Geometry: final body of the model. Coordinates: model frame, mm. A direction names the side the tool comes from. Round coordinates to 2 decimals unless told otherwise and drop trailing zeros. Loops run counter-clockwise (first coordinate to the right, second up) from the corner with the lowest first, then second, coordinate; pieces in that order, holes last. Notation, with made-up numbers: (75.25, 39.5) - (133.25, 39.5) arc R10 ccw to (133.25, 46.5) - close; hole circle Ø5 at (20, -5). An arc over 180 degrees is marked (long way). Return JSON: item names as keys, results as strings. Group by question number.
1. Draft query along X for faces 6 (the face through (20.4, 3.04, 12.43)), 7 (the face through (-6, -9, -17.5)), 8 (the face through (2.1, -14.2, -23.5)). Return one class per face: +X half, -X half, draft (parallel to the pull), parting line (faces both ways), or undercut.
2. Section B-B on z = 26.5. Return loops of the section in (x, y).
3. Material intervals for probe 1 along X at (y, z) = (-14.35, 26.5); probe 2 along X at (y, z) = (0.65, 8); probe 3 along Z at (x, y) = (1, -12), sorted ascending.
4. Section A-A on x = 17.5. Return loops of the section in (y, z).
5. Section C-C on x = 2. Count the separate pieces of the cut face and the enclosed holes in it, and give its area (3 significant figures).
6. First-contact query: pin 1 Ø11.5 at (x, y) = (-21, 15.5) entering from -Z; pin 2 Ø15.5 at (x, z) = (10.5, 2.5) entering from +Y; pin 3 Ø11 at (y, z) = (2.5, -8) entering from -X. Flat tips, straight axial feed; report the tip coordinate or a pass-through.
7. Set-up query: faces 1 (the face through (-6, -6, -20.5)), 2 (the face through (-6, -6, 20.5)), 3 (the face through (-13, 7, 0)), 4 (the face through (-16, -15.25, 26)), 5 (the face through (-31.275, 56.945, 8.709)). Return all of +Z, -Z, +X, -X, +Y, -Y with unobstructed straight access to the full face (end or side cutting, diameter ignored); none if empty.
from build123d import *

# Parameters (mm, degrees)
SKETCH_1_W              = 42
SKETCH_1_H              = 26
SKETCH_1_R              = 1.7
EXTRUDE_1_DEPTH         = 6
SKETCH_15_W             = 6
SKETCH_15_H             = 26
EXTRUDE_4_DEPTH         = 15
EXTRUDE_5_DEPTH         = 26
SKETCH_17_W             = 36
SKETCH_17_H             = 36
SKETCH_17_R             = 1.6
EXTRUDE_6_DEPTH         = 5.638155725
FILLET_3_R              = 2
SKETCH_18_R             = 3
CUT_EXTRUDE_4_DEPTH     = 3
SKETCH_19_R             = 3
CUT_EXTRUDE_5_DEPTH     = 3
FILLET_4_R              = 1
FILLET_6_R              = 5
EXTRUDE_7_DEPTH         = 2
FILLET_7_R              = 5
FILLET_8_R              = 5
SKETCH_21_W             = 30
SKETCH_21_H             = 7.5
EXTRUDE_8_DEPTH         = 6
SKETCH_23_W             = 30
SKETCH_23_H             = 3
EXTRUDE_9_DEPTH         = 17.25
SKETCH_24_W             = 30
SKETCH_24_H             = 4
EXTRUDE_10_DEPTH        = 12
EXTRUDE_11_DEPTH        = 30
FILLET_9_R              = 2
CUT_EXTRUDE_6_DEPTH     = 38
FILLET_11_R             = 2
SKETCH_29_R             = 1.75
CUT_EXTRUDE_7_DEPTH     = 38
SKETCH_30_R             = 3
CUT_EXTRUDE_8_DEPTH     = 2
FILLET_9_OF_MIRROR_2_R  = 2
FILLET_11_OF_MIRROR_2_R = 2
FILLET_14_R             = 2


with BuildPart() as part:
    # 草图1 → 凸台-拉伸1 (new body)
    with BuildSketch(Plane(origin=(0, 0, 0), x_dir=(1, 0, 0), z_dir=(0, 1, 0))):
        Rectangle(SKETCH_1_W, SKETCH_1_H)
        with Locations(Location((17.5, 8, 0), (0, 0, 270))):
            Circle(SKETCH_1_R, mode=Mode.SUBTRACT)
        with Locations(Location((17.5, -8, 0), (0, 0, 90))):
            Circle(SKETCH_1_R, mode=Mode.SUBTRACT)
    extrude(amount=EXTRUDE_1_DEPTH)

    # 草图15 → 凸台-拉伸4 (add)
    with BuildSketch(Plane(origin=(0, 6, 0), x_dir=(1, 0, 0), z_dir=(0, 1, 0))):
        with Locations((-18, 0)):
            Rectangle(SKETCH_15_W, SKETCH_15_H)
    extrude(amount=EXTRUDE_4_DEPTH)

    # 草图16 → 凸台-拉伸5 (add)
    with BuildSketch(Plane.XY.offset(13)):
        Polygon((-15, 21), (-21.858229251, 39.842830003), (-27.15636258, 37.914467174), (-21, 21), align=None)
    extrude(amount=-EXTRUDE_5_DEPTH)

    # 草图17 → 凸台-拉伸6 (add)
    with BuildSketch(Plane(origin=(-11.794196751, -4.292736554, 0), x_dir=(0, 0, 1), z_dir=(-0.9396926207859104, -0.3420201433256632, 0))):
        with Locations((0, 62.915968046)):
            Rectangle(SKETCH_17_W, SKETCH_17_H)
        with Locations(Location((10, 62.915968046, 0), (0, 0, 270))):
            Circle(SKETCH_17_R, mode=Mode.SUBTRACT)
        with Locations(Location((-10, 62.915968046, 0), (0, 0, 90))):
            Circle(SKETCH_17_R, mode=Mode.SUBTRACT)
    extrude(amount=-EXTRUDE_6_DEPTH)

    # 圆角3
    fillet_3_edges = [part.edges().sort_by_distance(p)[0] for p in [
        (-24.507295915, 38.878648589, 13),
        (-24.507295915, 38.878648589, -13),
        (-24.507295915, 38.878648589, 18),
        (-36.820021075, 72.707582937, 18),
        (-24.507295915, 38.878648589, -18),
        (-36.820021075, 72.707582937, -18),
    ]]
    fillet(fillet_3_edges, radius=FILLET_3_R)

    # 草图18 → 切除-拉伸4 (cut)
    with BuildSketch(Plane(origin=(-6.496063422, -2.364373725, 0), x_dir=(0, 0, -1), z_dir=(0.9396926207859105, 0.34202014332566305, 0))):
        with Locations(Location((-10, 62.915968046, 0), (0, 0, 90))):
            Circle(SKETCH_18_R)
        with Locations(Location((10, 62.915968046, 0), (0, 0, 90))):
            Circle(SKETCH_18_R)
    extrude(amount=-CUT_EXTRUDE_4_DEPTH, mode=Mode.SUBTRACT)

    # 草图19 → 切除-拉伸5 (cut)
    with BuildSketch(Plane(origin=(0, 6, 0), x_dir=(1, 0, 0), z_dir=(0, 1, 0))):
        with Locations(Location((17.5, 8, 0), (0, 0, 270))):
            Circle(SKETCH_19_R)
        with Locations(Location((17.5, -8, 0), (0, 0, 270))):
            Circle(SKETCH_19_R)
    extrude(amount=-CUT_EXTRUDE_5_DEPTH, mode=Mode.SUBTRACT)

    # 圆角4
    fillet_4_edges = [part.edges().sort_by_distance(p)[0] for p in [
        (-15, 13.5, 13),
        (-15, 13.5, -13),
        (-18.087094482, 29.481722381, 13),
        (-18.087094482, 29.481722381, -13),
        (-21.85822925, 39.842830003, -15.5),
        (-21.85822925, 39.842830003, 15.5),
        (-28.01459183, 56.757297177, 18),
        (-34.17095441, 73.671764352, 0),
        (-28.01459183, 56.757297177, -18),
        (-33.970603649, 73.121305159, -17.414213562),
        (-22.058580012, 40.393289196, -17.414213562),
        (-22.058580012, 40.393289196, 17.414213562),
        (-33.970603649, 73.121305159, 17.414213562),
        (-21.657878489, 39.292370811, -13.585786438),
        (-21.657878489, 39.292370811, 13.585786438),
    ]]
    fillet(fillet_4_edges, radius=FILLET_4_R)

    # 圆角6
    # the kernel refuses this fillet: 5 mm, written as the material it adds along each edge
    with BuildSketch(Plane(origin=(-21, 21, 13), x_dir=(0, -1, 0), z_dir=(0, 0, -1))) as fillet_6_piece_1:
        with BuildLine():
            CenterArc((FILLET_6_R * 0.176326980708, FILLET_6_R), FILLET_6_R, 250, 20)
            Line((-FILLET_6_R * 0.165693162617, FILLET_6_R * 0.0603073792141), (0, 0))
            Line((0, 0), (FILLET_6_R * 0.176326980708, 0))
        make_face()
    extrude(amount=26)
    # the kernel refuses this fillet: 5 mm, written as the material it takes off along each edge
    with BuildSketch(Plane(origin=(-20, 20.118365097, -13), x_dir=(0.9396926207859104, 0.3420201433256632, 0), z_dir=(-0.3420201433256632, 0.9396926207859104, 0))) as fillet_6_2_piece_1:
        with BuildLine():
            CenterArc((4, -1), 1, 0, 90)
            Line((5, -1), (5, 0))
            Line((5, 0), (4, 0))
        make_face()
    revolve(axis=Axis((-20, 20.118365097, -13), (0, 0, -1)), revolution_arc=20, mode=Mode.SUBTRACT)
    with BuildSketch(Plane(origin=(-20, 20.118365097, 13), x_dir=(1, 0, 0), z_dir=(0, -1, 0))) as fillet_6_2_piece_2:
        with BuildLine():
            CenterArc((4, -1), 1, 0, 90)
            Line((5, -1), (5, 0))
            Line((5, 0), (4, 0))
        make_face()
    revolve(axis=Axis((-20, 20.118365097, 13), (0, 0, 1)), revolution_arc=20, mode=Mode.SUBTRACT)
    with BuildSketch(Plane(origin=(-15, 21.000000001, -13), x_dir=(-0.34202014332566494, 0.9396926207859098, 0), z_dir=(0, 0, 1))) as fillet_6_2_piece_3:
        with BuildLine():
            CenterArc((FILLET_6_R * 0.176326980708, FILLET_6_R), FILLET_6_R, 250, 20)
            Line((-FILLET_6_R * 0.165693162617, FILLET_6_R * 0.0603073792141), (0, 0))
            Line((0, 0), (FILLET_6_R * 0.176326980708, 0))
        make_face()
    extrude(amount=26, mode=Mode.SUBTRACT)

    # 草图20 → 凸台-拉伸7 (add, symmetric)
    with BuildSketch(Plane.XY.offset(8)):
        Polygon((-15, 16), (10, 6), (-15, 6), align=None)
    extrude_7 = extrude(amount=EXTRUDE_7_DEPTH, both=True)

    # 镜向1: 凸台-拉伸7 across plane
    add(extrude_7.mirror(Plane(origin=(0, 0, 0), x_dir=(1, 0, 0), z_dir=(0, 0, -1))))

    # 圆角7
    fillet_7_edges = [part.edges().sort_by_distance(p)[0] for p in [
        (-15, 16, 8),
        (10, 6, 8),
        (-15, 16, -8),
        (10, 6, -8),
    ]]
    fillet(fillet_7_edges, radius=FILLET_7_R)

    # 圆角8
    fillet_8_edges = [part.edges().sort_by_distance(p)[0] for p in [
        (-15, 6, 0),
    ]]
    fillet(fillet_8_edges, radius=FILLET_8_R)

    # 草图21 → 凸台-拉伸8 (add)
    with BuildSketch(Plane(origin=(0, 6, 0), x_dir=(1, 0, 0), z_dir=(0, 1, 0))):
        with Locations((-6, -16.75)):
            Rectangle(SKETCH_21_W, SKETCH_21_H)
    extrude_8 = extrude(amount=-EXTRUDE_8_DEPTH)

    # 草图23 → 凸台-拉伸9 (add)
    with BuildSketch(Plane.XZ):
        with Locations((-6, 19)):
            Rectangle(SKETCH_23_W, SKETCH_23_H)
    extrude_9 = extrude(amount=EXTRUDE_9_DEPTH)

    # 草图24 → 凸台-拉伸10 (add)
    with BuildSketch(Plane.XY.offset(20.5)):
        with Locations((-6, -15.25)):
            Rectangle(SKETCH_24_W, SKETCH_24_H)
    extrude_10 = extrude(amount=EXTRUDE_10_DEPTH)

    # 草图26 → 凸台-拉伸11 (add)
    with BuildSketch(Plane.ZY.offset(21)):
        with BuildLine():
            Line((17.5, -3.107864376), (17.5, 0))
            Line((17.5, 0), (14.446020213, 0))
            ThreePointArc((14.446020213, 0), (16.048419147, -1.4798306), (17.5, -3.107864376))
        make_face()
    extrude_11 = extrude(amount=-EXTRUDE_11_DEPTH)

    # 圆角9
    fillet_9_edges = [part.edges().sort_by_distance(p)[0] for p in [
        (-6, -3.107864376, 17.5),
        (-6, 0, 14.446020213),
    ]]
    fillet(fillet_9_edges, radius=FILLET_9_R)

    # 草图28 → 切除-拉伸6 (cut)
    with BuildSketch(Plane.ZY.offset(21)):
        with BuildLine():
            Line((20.5, 1.822231123), (20.5, 6))
            Line((20.5, 6), (15.602483777, 6))
            ThreePointArc((15.602483777, 6), (18.171702504, 4.052329171), (20.5, 1.822231123))
        make_face()
    cut_extrude_6 = extrude(amount=-CUT_EXTRUDE_6_DEPTH, mode=Mode.SUBTRACT)

    # 圆角11
    fillet_11_edges = [part.edges().sort_by_distance(p)[0] for p in [
        (-6, -17.25, 17.5),
        (-21, -15.25, 32.5),
        (9, -15.25, 32.5),
    ]]
    fillet(fillet_11_edges, radius=FILLET_11_R)

    # 草图29 → 切除-拉伸7 (cut)
    with BuildSketch(Plane(origin=(0, -13.25, 0), x_dir=(1, 0, 0), z_dir=(0, 1, 0))):
        with Locations(Location((2, -26.5, 0), (0, 0, 270))):
            Circle(SKETCH_29_R)
        with Locations(Location((-14, -26.5, 0), (0, 0, 270))):
            Circle(SKETCH_29_R)
    cut_extrude_7 = extrude(amount=-CUT_EXTRUDE_7_DEPTH, mode=Mode.SUBTRACT)

    # 草图30 → 切除-拉伸8 (cut)
    with BuildSketch(Plane(origin=(0, -13.25, 0), x_dir=(1, 0, 0), z_dir=(0, 1, 0))):
        with Locations(Location((2, -26.5, 0), (0, 0, 270))):
            Circle(SKETCH_30_R)
        with Locations(Location((-14, -26.5, 0), (0, 0, 270))):
            Circle(SKETCH_30_R)
    cut_extrude_8 = extrude(amount=-CUT_EXTRUDE_8_DEPTH, mode=Mode.SUBTRACT)

    # 镜向2: 凸台-拉伸8, 凸台-拉伸9, 凸台-拉伸10, 凸台-拉伸11, 切除-拉伸6, 切除-拉伸7, 切除-拉伸8 across plane
    add(extrude_8.mirror(Plane.XY))
    add(extrude_9.mirror(Plane.XY))
    add(extrude_10.mirror(Plane.XY))
    add(extrude_11.mirror(Plane.XY))
    add(cut_extrude_6.mirror(Plane.XY), mode=Mode.SUBTRACT)
    add(cut_extrude_7.mirror(Plane.XY), mode=Mode.SUBTRACT)
    add(cut_extrude_8.mirror(Plane.XY), mode=Mode.SUBTRACT)

    # 圆角9 of 镜向2
    fillet_9_of_mirror_2_edges = [part.edges().sort_by_distance(p)[0] for p in [
        (-6, -3.107864376, -17.5),
        (-6, 0, -14.446020213),
    ]]
    fillet(fillet_9_of_mirror_2_edges, radius=FILLET_9_OF_MIRROR_2_R)

    # 圆角11 of 镜向2
    fillet_11_of_mirror_2_edges = [part.edges().sort_by_distance(p)[0] for p in [
        (-6, -17.25, -17.5),
        (-21, -15.25, -32.5),
        (9, -15.25, -32.5),
    ]]
    fillet(fillet_11_of_mirror_2_edges, radius=FILLET_11_OF_MIRROR_2_R)

    # 圆角14
    fillet_14_edges = [part.edges().sort_by_distance(p)[0] for p in [
        (9, 3, 13),
        (9, 3, -13),
        (21, 3, 13),
        (21, 3, -13),
    ]]
    fillet(fillet_14_edges, radius=FILLET_14_R)


solid = part.part
Taken from the geometry:
{
 "1": {"face 6": "+X half", "face 7": "draft", "face 8": "undercut"},
 "2": {"outline": "(-21, -17.25) - (-15.75, -17.25) - (-15.75, -15.25) - (-17, -15.25) - (-17, -13.25) - (-21, -13.25) - close; (-12.25, -17.25) - (0.25, -17.25) - (0.25, -15.25) - (-1, -15.25) - (-1, -13.25) - (-11, -13.25) - (-11, -15.25) - (-12.25, -15.25) - close; (3.75, -17.25) - (9, -17.25) - (9, -13.25) - (5, -13.25) - (5, -15.25) - (3.75, -15.25) - close"},
 "3": {"probe 1": "-21 to -17, -11 to -1, 5 to 9", "probe 2": "-21 to 15.8, 19.2 to 21", "probe 3": "-20.5 to -17.5, 17.5 to 20.5"},
 "4": {"outline": "(0, -13) - (6, -13) - (6, -11) - (3, -11) - (3, -9.7) - (0, -9.7) - close; (0, -6.3) - (3, -6.3) - (3, -5) - (6, -5) - (6, 5) - (3, 5) - (3, 6.3) - (0, 6.3) - close; (0, 9.7) - (3, 9.7) - (3, 11) - (6, 11) - (6, 13) - (0, 13) - close"},
 "5": {"separate pieces": "3", "enclosed holes": "0", "area": "422 mm2"},
 "6": {"pin 1": "z = -13", "pin 2": "y = 8.57", "pin 3": "x = -21"},
 "7": {"face 1": "-Z, +X, -X, +Y", "face 2": "+Z, +X, -X, +Y", "face 3": "+X, +Y", "face 4": "+Y", "face 5": "none"}
}
